from build123d import *

# Parameters (mm, degrees)
SKETCH2_W           = 100
SKETCH2_H           = 75
SKETCH2_R           = 6
BOSS_EXTRUDE1_DEPTH = 5
SKETCH3_W           = 100
SKETCH3_H           = 10
BOSS_EXTRUDE2_DEPTH = 50
CUT_EXTRUDE2_START  = -10
CUT_EXTRUDE2_DEPTH  = 10
FILLET1_R           = 1
FILLET2_R           = 1
SKETCH6_R           = 7.5
BOSS_EXTRUDE3_DEPTH = 90


# Read off the part's stored shape, not the designer's step: Cut-Extrude2
with BuildPart() as part:
    # Sketch2 → Boss-Extrude1 (new body)
    with BuildSketch(Plane(origin=(0, 0, 0), x_dir=(1, 0, 0), z_dir=(0, 1, 0))):
        Rectangle(SKETCH2_W, SKETCH2_H)
        with Locations(Location((-32, -22.5, 0), (0, 0, 270))):
            Circle(SKETCH2_R, mode=Mode.SUBTRACT)
        with Locations(Location((32, -22.5, 0), (0, 0, 270))):
            Circle(SKETCH2_R, mode=Mode.SUBTRACT)
    extrude(amount=BOSS_EXTRUDE1_DEPTH)

    # Sketch3 → Boss-Extrude2 (add)
    with BuildSketch(Plane(origin=(0, 5, 0), x_dir=(1, 0, 0), z_dir=(0, 1, 0))):
        with Locations((0, 32.5)):
            Rectangle(SKETCH3_W, SKETCH3_H)
    extrude(amount=BOSS_EXTRUDE2_DEPTH)

    # Cut-Extrude2 outline → Cut-Extrude2 (cut)
    with BuildSketch(Plane.XY.offset(-27.5).offset(CUT_EXTRUDE2_START)):
        with BuildLine():
            Line((-50, 55), (-50, 5))
            ThreePointArc((-50, 5), (-35.355339097, 40.355339022), (-1.05e-07, 55))
            Line((-1.05e-07, 55), (-50, 55))
        make_face()
        with BuildLine():
            Line((50, 55), (-1.05e-07, 55))
            ThreePointArc((-1.05e-07, 55), (35.355339022, 40.355339097), (50, 5))
            Line((50, 5), (50, 55))
        make_face()
    extrude(amount=CUT_EXTRUDE2_DEPTH, mode=Mode.SUBTRACT)

    # Fillet1
    fillet1_edges = [part.edges().sort_by_distance(p)[0] for p in [
        (-50, 2.5, -37.5),
        (50, 2.5, -37.5),
        (35.355339022, 40.355339097, -37.5),
    ]]
    fillet(fillet1_edges, radius=FILLET1_R)

    # Fillet2
    fillet2_edges = [part.edges().sort_by_distance(p)[0] for p in [
        (35.355339022, 40.355339097, -27.5),
    ]]
    fillet(fillet2_edges, radius=FILLET2_R)

    # Sketch6 → Boss-Extrude3 (add)
    with BuildSketch(Plane.XY.offset(-27.5)):
        with Locations((0, 27)):
            Circle(SKETCH6_R)
    extrude(amount=-BOSS_EXTRUDE3_DEPTH)


solid = part.part
Input: part model. Units: mm. Frame: model coordinates. A direction names the side the tool comes from. Coordinates: 2 decimals unless noted, no trailing zeros. Loops run counter-clockwise (first coordinate to the right, second up) from the corner with the lowest first, then second, coordinate; pieces in that order, holes last. Notation, with made-up numbers: (-5.75, 18) - (9.25, 18) arc R25 ccw to (9.25, 35) - close; hole circle Ø4 at (-21, 25.25). An arc over 180 degrees is marked (long way). Answer in a Markdown table with one row per item. Add a question column.
Item 1: Mould query, pull axis Y, two halves, no side actions, for faces 1 (the flat face through (-1, 2, 37.5)), 2 (the cylindrical face through (-0.976, 34.436, -76.94)), 3 (the flat face through (-1, 0, -1)), 4 (the flat face through (-1, 5, 4)). Classes: released by +Y, released by -Y, zero draft, split by the parting line, or undercut.
Item 2: Line query: line 1 along X through (y, z) = (1, 22); line 2 along Z through (x, y) = (-3.5, 33); line 3 along Z through (x, y) = (-16, 18). Output: solid intervals per line, ascending. Write a range as [from, to].
Item 3: Section query A-A on z = -86.5. Return the cut outline in (x, y).
Item 4: Access query for faces 5 (the flat face through (-1, 24, -27.5)), 6 (the flat face through (-50, 2, 1)). Directions: +Z, -Z, +X, -X, +Y, -Y. A direction counts if a zero-diameter tool reaches every point of the face in a straight line with its end or side. Return the directions, or none.
Item 5: Contact query for flat-ended pins moving along their axis: P1, Ø5, axis at x = -4, z = -28.5, coming from the +Y side; P2, Ø2, axis at x = 12.5, y = 27, coming from the +Z side; P3, Ø5, axis at x = 25, z = -21.5, coming from the -Y side; P4, Ø3, axis at y = 32.5, z = -27, coming from the -X side. Output: stop coordinate, or through.
Item 6: Section query B-B on z = -23. Return the cut outline in (x, y).
Recorded:
| question | item | result |
|---|---|---|
| 1 | face 1 | zero draft |
| 1 | face 2 | split by the parting line |
| 1 | face 3 | released by -Y |
| 1 | face 4 | released by +Y |
| 2 | line 1 | [-50, -37.98], [-26.02, 26.02], [37.98, 50] |
| 2 | line 2 | [-117.5, -27.5] |
| 2 | line 3 | [-37.5, -27.5] |
| 3 | outline | circle Ø15 at (0, 27) |
| 4 | face 5 | +Z, +X, -X, +Y |
| 4 | face 6 | +Z, -Z, -X, +Y, -Y |
| 5 | P1 | y = 54.98 |
| 5 | P2 | z = -27.5 |
| 5 | P3 | y = 0 |
| 5 | P4 | x = -42.32 |
| 6 | outline | (-50, 0) - (50, 0) - (50, 5) - (-50, 5) - close |
